Autodesk Inventor part; units mm, degrees
ref_plane "YZ Plane" through (0, 0, 0) normal (1, 0, 0) x (0, 1, 0)
ref_plane "XZ Plane" through (0, 0, 0) normal (0, 1, 0) x (-1, 0, 0)
ref_plane "XY Plane" through (0, 0, 0) normal (0, 0, 1) x (1, 0, 0)
sketch "Sketch1" plane through (0, 0, 0) normal (0, 0, 1) x (1, 0, 0)
  line L0 (0, 0) -> (2, 0)
  line L1 (2, 0) -> (2, 16)
  line L2 (2, 16) -> (0, 16)
  line L3 (0, 16) -> (0, 0)
  line L4 (2, 2) -> (8, 2)
  line L5 (8, 2) -> (8, 0)
  line L6 (8, 0) -> (2, 0)
  line L7 (2, 0) -> (2, 2)
  dimension "d0" = 2
  dimension "d1" = 16
  dimension "d2" = 6
extrude "Extrusion1" add sketch "Sketch1" against normal blind 22
sketch "Sketch3" plane through (2, 2, 0) normal (1, 0, 0) x (0, 0, -1)
  line L0 (9.5, 14) -> (4.5, 14)
  line L1 (4.5, 14) -> (4.5, 8)
  line L2 (4.5, 8) -> (9.5, 8)
  line L3 (9.5, 8) -> (9.5, 14)
  point P0 (0, -2)
  dimension "d9" = 5
  dimension "d10" = 6
extrude "Extrusion3" cut sketch "Sketch3" against normal blind 10
fillet "Fillet1" radius 0.8 7 edges at (2, 10, -7) (0, 10, -7) (1, 16, -9.5) (2, 13, -9.5) (0, 13, -9.5) (2, 13, -4.5) (0, 13, -4.5)
properties part number "housing_mate_v07"
The model under review builds one solid part; all positions refer to its coordinate system, in mm. A direction names the side the tool comes from. Coordinates: 2 decimals unless noted, no trailing zeros. Write each loop counter-clockwise with the first axis right and the second up, starting at its lowest first coordinate (ties: lowest second). Pieces come first, ordered by that corner, then holes. Notation, with made-up numbers: (-16, -16) - (35, -16) arc R21 cw to (35, -9) - close; hole circle Ø11 at (86.5, 51.5). An arc over 180 degrees is marked (long way). Answer as a JSON object with one key per item and string values. Group by question number.
1. Machinability: for faces 4 (the face through (2, 9, -11)), 5 (the face through (0.24, 12.65, -4.27)), 6 (the face through (1.76, 12.55, -4.27)), which of the approach directions +Z, -Z, +X, -X, +Y, -Y give a long, thin tool a straight path to every point of the face, cutting with its end or side? Answer none if there is none.
2. Add section C-C (x = 5). Give the boundary of the cut face in (y, z), plus the area to 3 significant figures.
3. Clearance check with flat-ended pins moving along their axes: pin 1 Ø1.5 at (x, z) = (6.5, -13.5) entering from +Y; pin 2 Ø5 at (y, z) = (8.5, -19) entering from +X. State where each tip first meets the part, or that it passes through.
4. Mouldability with a two-part tool opening along Z and no side actions: class faces 1 (the face through (8, 1, -11)), 2 (the face through (1.6, 5.7, -22)), 3 (the face through (0.24, 12.55, -9.73)) as pulls with the +Z half, pulls with the -Z half, needs draft (parallel to the pull), parting line crosses it, or undercut.
5. To check wall thickness, follow probe 1 along Z at (x, y) = (1.25, 12.75); probe 2 along Y at (x, z) = (3, -14.5). State the ranges of each line that lie inside material, in increasing order.
6. Add section B-B (z = -8.25). Give the boundary of the cut face in (x, y).
7. Add section A-A (y = 13.5). Give the boundary of the cut face in (x, z), plus the area to 3 significant figures.
Findings:
{
 "1": {"face 4": "+Z, -Z, +X, +Y", "face 5": "-X, +Y", "face 6": "+X, +Y"},
 "2": {"outline": "(0, -22) - (2, -22) - (2, 0) - (0, 0) - close", "area": "44.0 mm²"},
 "3": {"pin 1": "y = 2", "pin 2": "x = 2"},
 "4": {"face 1": "needs draft", "face 2": "pulls with the -Z half", "face 3": "undercut"},
 "5": {"probe 1": "-22 to -9.5, -4.5 to 0", "probe 2": "0 to 2"},
 "6": {"outline": "(0, 0) - (8, 0) - (8, 2) - (2, 2) - (2, 9.2) arc R0.8 ccw to (1.2, 10) - (0.8, 10) arc R0.8 ccw to (0, 9.2) - close"},
 "7": {"outline": "(0, -22) - (2, -22) - (2, -10.3) arc R0.8 ccw to (1.2, -9.5) - (0.8, -9.5) arc R0.8 ccw to (0, -10.3) - close; (0, -3.7) arc R0.8 ccw to (0.8, -4.5) - (1.2, -4.5) arc R0.8 ccw to (2, -3.7) - (2, 0) - (0, 0) - close", "area": "33.5 mm²"}
}
